Autodesk Inventor part; units mm, degrees
ref_plane "YZ Plane" through (0, 0, 0) normal (1, 0, 0) x (0, 1, 0)
sketch "Sketch2" plane through (0, 0, 0) normal (0, 0, 1) x (1, 0, 0)
  line L0 (-25.4, -19.05) -> (25.4, -19.05)
  line L1 (25.4, -19.05) -> (25.4, 19.05)
  line L2 (25.4, 19.05) -> (-25.4, 19.05)
  line L3 (-25.4, 19.05) -> (-25.4, -19.05)
  line L4 (-25.4, -19.05) -> (25.4, 19.05) construction
  line L5 (25.4, -19.05) -> (-25.4, 19.05) construction
  point P0 (0, 0)
  dimension "d4" = 50.8
  dimension "d5" = 38.1
extrude "Extrusion2" add sketch "Sketch2" along normal mid plane 38.1
sketch "Sketch3" plane through (-25.4, 19.05, 19.05) normal (0, 1, 0) x (1, 0, 0)
  line L0 (0, 0) -> (0, 38.1) construction
  line L1 (38.1, 19.05) -> (38.1, 25.908)
  line L2 (38.1, 25.908) -> (0, 25.908)
  line L3 (0, 25.908) -> (0, 19.05)
  line L4 (0, 0) -> (0, 25.4) construction
  line L5 (38.1, 19.05) -> (38.1, 12.192)
  line L6 (38.1, 12.192) -> (0, 12.192)
  line L7 (0, 12.192) -> (0, 19.05)
  line L8 (50.8, 0) -> (0, 0)
  point P0 (25.4, 19.05)
  dimension "d8" = 38.1
  dimension "d10" = 13.716
  dimension "d34" = 12.192
extrude "Extrusion3" cut sketch "Sketch3" against normal through all
sketch "Sketch4" plane through (0, 0, 19.05) normal (0, 0, 1) x (1, 0, 0)
  circle A0 centre (-12.7, 0) radius 5.2705
  line L0 (-25.4, 19.05) -> (-25.4, -19.05)
  point P0 (0, 0)
  dimension "d13" = 10.541
  dimension "d14" = 12.7
extrude "Extrusion4" cut sketch "Sketch4" against normal through all
sketch "Sketch5" plane through (25.4, -19.05, 19.05) normal (1, 0, 0) x (0, 0, -1)
  circle A0 centre (19.05, 19.05) radius 4.2164
  dimension "d27" = 8.4328
extrude "Extrusion5" cut sketch "Sketch5" against normal blind 12.7
properties part number "pistonFor-8-in" material "PET Plastic"
Work out the finished part from the listing and answer in its coordinate system (mm). A direction names the side the tool comes from. Give positions to 0.01 mm unless a question says otherwise; leave off trailing zeros. Loops run counter-clockwise (first coordinate to the right, second up) from the corner with the lowest first, then second, coordinate; pieces in that order, holes last. Notation, with made-up numbers: (0, 17.25) -> (44, 17.25) arc R21 ccw to (44, 22.25) -> close; hole circle Ø2 at (39, 87). An arc over 180 degrees is marked (long way). Write item = value, one per line. Start each with the question number.
(1) Which of the six approach directions +Z, -Z, +X, -X, +Y, -Y give full straight-line access (tool end or side, diameter ignored) to faces 5 (the flat face through (-25.4, 0, 13)), 6 (the flat face through (-6, 0, -6.858))?
(2) Find section D-D on x = 4. Give the vertices of the cut face in (y, z), and give its area (3 significant figures).
(3) Find section B-B on y = 0. Give the vertices of the cut face in (x, z), and give its area (3 significant figures).
(4) The mould has two halves that part along Z. Classify faces 1 (the flat face through (12.7, 5, 0)), 2 (the flat face through (0, 0, -19.05)), 3 (the flat face through (0, 0, 19.05)), 4 (the flat face through (25.4, 0, -5)): +Z half, -Z half, draft (parallel to the pull), parting line (faces both ways), or undercut.
(5) Find section C-C on z = 0. Give the vertices of the cut face in (x, y).
(6) Find the intervals of material crossed by probe 1 along Z at (x, y) = (4.5, -14); probe 2 along Y at (x, z) = (-12.7, -13.25); probe 3 along Y at (x, z) = (16.75, 0), in increasing order. Write a range as from..to.
(7) Given pin 1 Ø1 at (y, z) = (7.5, -5.5) entering from -X, flat-ended and moving along its own axis, determine where the tip first touches the part or whether it passes through.
(8) Find section A-A on x = -12.7. Give the vertices of the cut face in (y, z).
From the geometry:
q1.face_5 = +Z, -Z, -X, +Y, -Y
q1.face_6 = -X, +Y, -Y
q2.outline = (-19.05, -19.05) -> (19.05, -19.05) -> (19.05, -6.86) -> (-19.05, -6.86) -> close; (-19.05, 6.86) -> (19.05, 6.86) -> (19.05, 19.05) -> (-19.05, 19.05) -> close
q2.area = 929 mm^2
q3.outline = (-25.4, -19.05) -> (-17.97, -19.05) -> (-17.97, -6.86) -> (-25.4, -6.86) -> close; (-25.4, 6.86) -> (-17.97, 6.86) -> (-17.97, 19.05) -> (-25.4, 19.05) -> close; (-7.43, -19.05) -> (25.4, -19.05) -> (25.4, -4.22) -> (12.7, -4.22) -> (12.7, -6.86) -> (-7.43, -6.86) -> close; (-7.43, 6.86) -> (12.7, 6.86) -> (12.7, 4.22) -> (25.4, 4.22) -> (25.4, 19.05) -> (-7.43, 19.05) -> close
q3.area = 1,050 mm^2
q4.face_1 = undercut
q4.face_2 = -Z half
q4.face_3 = +Z half
q4.face_4 = draft
q5.outline = (12.7, -19.05) -> (25.4, -19.05) -> (25.4, -4.22) -> (12.7, -4.22) -> close; (12.7, 4.22) -> (25.4, 4.22) -> (25.4, 19.05) -> (12.7, 19.05) -> close
q6.probe_1 = -19.05..-6.86, 6.86..19.05
q6.probe_2 = -19.05..-5.27, 5.27..19.05
q6.probe_3 = -19.05..-4.22, 4.22..19.05
q7.pin_1 = 12.7
q8.outline = (-19.05, -19.05) -> (-5.27, -19.05) -> (-5.27, -6.86) -> (-19.05, -6.86) -> close; (-19.05, 6.86) -> (-5.27, 6.86) -> (-5.27, 19.05) -> (-19.05, 19.05) -> close; (5.27, -19.05) -> (19.05, -19.05) -> (19.05, -6.86) -> (5.27, -6.86) -> close; (5.27, 6.86) -> (19.05, 6.86) -> (19.05, 19.05) -> (5.27, 19.05) -> close
